Build history of the part. All positions in model axes, mm. Round coordinates to 2 decimals unless told otherwise and drop trailing zeros. Loops run counter-clockwise (first coordinate to the right, second up) from the corner with the lowest first, then second, coordinate; pieces in that order, holes last. Notation, with made-up numbers: (32, -0.5) - (70, -0.5) arc R34 cw to (70, 29.5) - close; hole circle Ø11 at (38.25, -20.75). An arc over 180 degrees is marked (long way). Answer as CSV lines item,"result". Start each with the question number.
```python
from build123d import *

# Parameters (mm, degrees)
SKETCH1_W           = 235.6
SKETCH1_H           = 290.9
BOSS_EXTRUDE1_DEPTH = 3.5
BOSS_EXTRUDE2_DEPTH = 3.5
SKETCH4_R           = 2
CUT_EXTRUDE1_DEPTH  = 3.5
SKETCH5_W           = 92.8
SKETCH5_H           = 120.45
CUT_EXTRUDE2_DEPTH  = 10
FILLET1_R           = 10


with BuildPart() as part:
    # Sketch1 → Boss-Extrude1 (new body)
    with BuildSketch(Plane(origin=(0, 0, 0), x_dir=(1, 0, 0), z_dir=(0, 1, 0))):
        Rectangle(SKETCH1_W, SKETCH1_H)
    extrude(amount=BOSS_EXTRUDE1_DEPTH)

    # Sketch3 → Boss-Extrude2 (add)
    with BuildSketch(Plane(origin=(0, 3.5, 0), x_dir=(1, 0, 0), z_dir=(0, 1, 0))):
        with BuildLine():
            Line((-20, -145.45), (20, -145.45))
            ThreePointArc((20, -145.45), (0, -165.45), (-20, -145.45))
        make_face()
    extrude(amount=-BOSS_EXTRUDE2_DEPTH)

    # Sketch4 → Cut-Extrude1 (cut)
    with BuildSketch(Plane(origin=(0, 3.5, 0), x_dir=(1, 0, 0), z_dir=(0, 1, 0))):
        with Locations(Location((0, -160.45, 0), (0, 0, 270))):
            Circle(SKETCH4_R)
    extrude(amount=-CUT_EXTRUDE1_DEPTH, mode=Mode.SUBTRACT)

    # Sketch5 → Cut-Extrude2 (cut)
    with BuildSketch(Plane(origin=(0, 3.5, 0), x_dir=(1, 0, 0), z_dir=(0, 1, 0))):
        with Locations((-56.4, 70.225)):
            Rectangle(SKETCH5_W, SKETCH5_H)
        with Locations((56.4, 70.225)):
            Rectangle(SKETCH5_W, SKETCH5_H)
        with Locations((-56.4, -70.225)):
            Rectangle(SKETCH5_W, SKETCH5_H)
        with Locations((56.4, -70.225)):
            Rectangle(SKETCH5_W, SKETCH5_H)
    extrude(amount=-CUT_EXTRUDE2_DEPTH, mode=Mode.SUBTRACT)

    # Fillet1
    fillet1_edges = [part.edges().sort_by_distance(p)[0] for p in [
        (10, 1.75, -10),
        (10, 1.75, -130.45),
        (102.8, 1.75, -130.45),
        (102.8, 1.75, -10),
        (-102.8, 1.75, 130.45),
        (-102.8, 1.75, 10),
        (-10, 1.75, 10),
        (-10, 1.75, 130.45),
        (10, 1.75, 130.45),
        (10, 1.75, 10),
        (102.8, 1.75, 10),
        (102.8, 1.75, 130.45),
        (-102.8, 1.75, -10),
        (-102.8, 1.75, -130.45),
        (-10, 1.75, -130.45),
        (-10, 1.75, -10),
    ]]
    fillet(fillet1_edges, radius=FILLET1_R)


solid = part.part
```
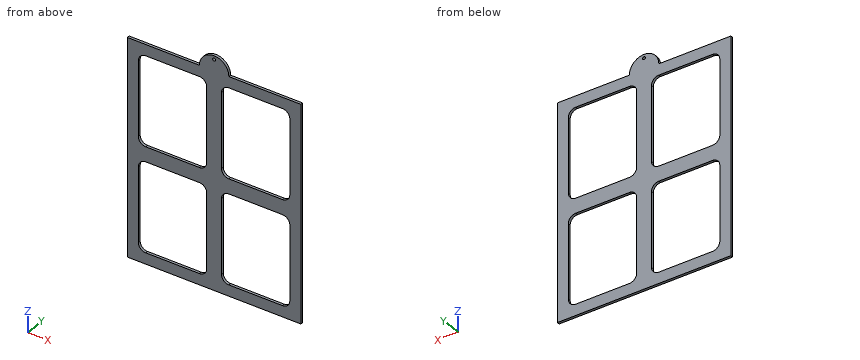
Q1. Band-saw the part on C-C, the plane y = 1.85. Give the number of separate pieces and of enclosed holes in the cut face, then the cut area to 3 significant figures.
Q2. Band-saw the part on B-B, the plane x = 66. List the corners of the cut face in (y, z).
Q3. Wall check: probe 1 along Z at (x, y) = (-71.5, 0.5); probe 2 along X at (y, z) = (0.8, -22.5); probe 3 along Z at (x, y) = (-14.5, 2.1). Give the ranges that are in metal, low to high. Write a range as [from, to].
Q4. Band-saw the part on A-A, the plane z = 37. List the corners of the cut face in (x, y).
Q5. Pin check, flat tips, straight feed: pin 1 Ø1 at (x, y) = (67.5, 2) entering from +Z; pin 2 Ø3 at (x, z) = (-11, 128.5) entering from -Y. Stop position of each tip, or through.
Reported:
1,separate pieces,"1"
1,enclosed holes,"5"
1,area,"24,800 mm2"
2,outline,"(0, -145.45) - (3.5, -145.45) - (3.5, -130.45) - (0, -130.45) - close; (0, -10) - (3.5, -10) - (3.5, 10) - (0, 10) - close; (0, 130.45) - (3.5, 130.45) - (3.5, 145.45) - (0, 145.45) - close"
3,probe 1,"z = [-145.45, -130.45], [-10, 10], [130.45, 145.45]"
3,probe 2,"x = [-117.8, -102.8], [-10, 10], [102.8, 117.8]"
3,probe 3,"z = [-145.45, -128.8], [-11.65, 11.65], [128.8, 159.22]"
4,outline,"(-117.8, 0) - (-102.8, 0) - (-102.8, 3.5) - (-117.8, 3.5) - close; (-10, 0) - (10, 0) - (10, 3.5) - (-10, 3.5) - close; (102.8, 0) - (117.8, 0) - (117.8, 3.5) - (102.8, 3.5) - close"
5,pin 1,"stops at z = 145.45"
5,pin 2,"stops at y = 0"
